CAD build for the part. Positions are in the model's coordinates, mm. A direction names the side the tool comes from. Round coordinates to 2 decimals unless told otherwise and drop trailing zeros. Order: outer loops, then holes, each group sorted by start corner. A loop starts at its lowest first (then second) coordinate and runs counter-clockwise, first axis right, second up. Notation, with made-up numbers: M -27.75,28 L 16.25,28 A17 cw 16.25,61 Z; hole C 67.5,85.25 d6. An arc over 180 degrees is marked long. Put each result on its own line as item: value.
```python
from build123d import *

# Parameters (mm, degrees)
F0_R     = 19.05
F1_DEPTH = 76.2
F2_R     = 19.05
F3_DEPTH = 20.32
F4_DEPTH = 76.2
F5_D     = 33.02
F5_DEPTH = 20.321
F6_D     = 33.02
F7_D     = 33.02
F7_DEPTH = 76.201
F8_D     = 33.02


with BuildPart() as f1:
    # F0 (on Front) → F1 (new body)
    with BuildSketch(Plane.XZ):
        Circle(F0_R)
    extrude(amount=F1_DEPTH)

    # F2 (on Right) → F3 (join, symmetric)
    with BuildSketch(Plane.YZ):
        Circle(F2_R)
    extrude(amount=F3_DEPTH, both=True)

    # F0 (on Front) → F4 (join)
    with BuildSketch(Plane.XZ):
        Circle(F0_R)
    extrude(amount=-F4_DEPTH)

    # F5 (through all, one way)
    with BuildSketch(Plane(origin=(0, 0, 0), x_dir=(0, 1, 0), z_dir=(-1, 0, 0))):
        with Locations((0, 0)):
            Circle(F5_D / 2)
    extrude(amount=-F5_DEPTH, mode=Mode.SUBTRACT)

    # F6 (through all)
    with Locations(Plane.YZ):
        with Locations((0, 0)):
            Hole(F6_D / 2)

    # F7 (through all, one way)
    with BuildSketch(Plane(origin=(0, 0, 0), x_dir=(1, 0, 0), z_dir=(0, 1, 0))):
        with Locations((0, 0)):
            Circle(F7_D / 2)
    extrude(amount=-F7_DEPTH, mode=Mode.SUBTRACT)

    # F8 (through all)
    with Locations(Plane.XZ):
        with Locations((0, 0)):
            Hole(F8_D / 2)


solid = f1.part
```
Item 1: Band-saw the part on D-D on z = -10. Give the cut face in (x, y).
Answers below:
outline: M -20.32,-16.21 L -16.21,-16.21 L -16.21,-76.2 L -13.14,-76.2 L -13.14,-13.14 L -20.32,-13.14 Z; M -20.32,13.14 L -13.14,13.14 L -13.14,76.2 L -16.21,76.2 L -16.21,16.21 L -20.32,16.21 Z; M 13.14,-76.2 L 16.21,-76.2 L 16.21,-16.21 L 20.32,-16.21 L 20.32,-13.14 L 13.14,-13.14 Z; M 13.14,13.14 L 20.32,13.14 L 20.32,16.21 L 16.21,16.21 L 16.21,76.2 L 13.14,76.2 Z
Item 2: Band-saw the part on A-A on z = 0. Give the cut face in (x, y).
Answers below:
outline: M -20.32,-19.05 L -19.05,-19.05 L -19.05,-76.2 L -16.51,-76.2 L -16.51,-16.51 L -20.32,-16.51 Z; M -20.32,16.51 L -16.51,16.51 L -16.51,76.2 L -19.05,76.2 L -19.05,19.05 L -20.32,19.05 Z; M 16.51,-76.2 L 19.05,-76.2 L 19.05,-19.05 L 20.32,-19.05 L 20.32,-16.51 L 16.51,-16.51 Z; M 16.51,16.51 L 20.32,16.51 L 20.32,19.05 L 19.05,19.05 L 19.05,76.2 L 16.51,76.2 Z
Item 3: Pin check, flat tips, straight feed: P1, Ø3, axis at x = -12.5, y = -5.5, coming from the -Z side; P2, Ø12, axis at y = 51, z = 1, coming from the -X side; P3, Ø6, axis at x = 8, y = -32, coming from the +Z side; P4, Ø10, axis at x = -3, z = -7, coming from the -Y side. Stop position of each tip, or through.
Answers below:
P1: z = -18.63
P2: x = -19.05
P3: z = 18.38
P4: through
Item 4: Mould opens along Z. For faces 1 (the cylindrical face through (14.818, -2.48, 18.888)), 2 (the cylindrical face through (14.533, -12.169, -11.158)), 3 (the flat face through (-6, 76.2, 16)) say: pulls with the +Z half, pulls with the -Z half, needs draft (parallel to the pull), parting line crosses it, or undercut.
Answers below:
face 1: parting line crosses it
face 2: undercut
face 3: needs draft
Item 5: Band-saw the part on B-B on x = -9. Give the cut face in (y, z).
Answers below:
outline: M -76.2,-16.79 L -9,-16.79 A19.05 ccw 9,-16.79 L 76.2,-16.79 L 76.2,-13.84 L 9,-13.84 A16.51 cw -9,-13.84 L -76.2,-13.84 Z; M -76.2,13.84 L -9,13.84 A16.51 cw 9,13.84 L 76.2,13.84 L 76.2,16.79 L 9,16.79 A19.05 ccw -9,16.79 L -76.2,16.79 Z
Item 6: Probe line 1 along X through (y, z) = (-19, 0); line 2 along Z through (x, y) = (-0.5, 26); line 3 along Y through (x, z) = (-17, -1). List the from-to ranges inside material, lowest first. Write a range as [from, to].
Answers below:
line 1: [-20.32, -16.51], [16.51, 20.32]
line 2: [-19.04, -16.5], [16.5, 19.04]
line 3: [-76.2, -16.48], [16.48, 76.2]
Item 7: Band-saw the part on C-C on y = 31.5. Give the cut face in (x, z).
Answers below:
outline: C 0,0 d38.1; hole C 0,0 d33.02
Item 8: Tool access for faces 4 (the cylindrical face through (10.241, -46.033, 16.063)), 5 (the cylindrical face through (10.241, 46.033, 16.063)), 6 (the cylindrical face through (16.494, 47.1, 0.726)), 7 (the flat face through (20.32, -6, 16)), 8 (the cylindrical face through (-14.533, -14.041, 12.875)): list every direction of +Z, -Z, +X, -X, +Y, -Y with a clear straight run to the whole face (end or side of a thin tool).
Answers below:
face 4: -Y
face 5: +Y
face 6: +Y, -Y
face 7: +Z, -Z, +X, +Y, -Y
face 8: -X
